Build history of the part. All positions in model axes, mm. Face numbers are marked on the shaded views. A direction names the side the tool comes from. Coordinates: 2 decimals unless noted, no trailing zeros. Order: outer loops, then holes, each group sorted by start corner. A loop starts at its lowest first (then second) coordinate and runs counter-clockwise, first axis right, second up. Notation, with made-up numbers: (80.5, -14.75) - (111.5, -14.75) arc R20 cw to (111.5, 16.25) - close; hole circle Ø4 at (-38, -27.5). An arc over 180 degrees is marked (long way). Answer as CSV lines item,"result". Start each with the question number.
from build123d import *

# Parameters (mm, degrees)
SKETCH1_R           = 8
BOSS_EXTRUDE1_DEPTH = 25
SKETCH2_R           = 5.5
CUT_EXTRUDE1_DEPTH  = 20
SKETCH3_R           = 2.5
CUT_EXTRUDE2_DEPTH  = 6
FILLET1_R           = 0.2
FILLET2_R           = 0.3


with BuildPart() as part:
    # Sketch1 → Boss-Extrude1 (new body)
    with BuildSketch(Plane.XY):
        Circle(SKETCH1_R)
    extrude(amount=BOSS_EXTRUDE1_DEPTH)

    # Sketch2 → Cut-Extrude1 (cut)
    with BuildSketch(Plane.XY.offset(25)):
        Circle(SKETCH2_R)
    extrude(amount=-CUT_EXTRUDE1_DEPTH, mode=Mode.SUBTRACT)

    # Sketch3 → Cut-Extrude2 (cut, through all)
    with BuildSketch(Plane.XY.offset(5)):
        Circle(SKETCH3_R)
    extrude(amount=-CUT_EXTRUDE2_DEPTH, mode=Mode.SUBTRACT)

    # Fillet1
    fillet1_edges = [part.edges().sort_by_distance(p)[0] for p in [
        (-2.5, 0, 0),
        (-2.5, 0, 5),
        (-8, 0, 25),
        (-5.5, 0, 25),
    ]]
    fillet(fillet1_edges, radius=FILLET1_R)

    # Fillet2
    fillet2_edges = [part.edges().sort_by_distance(p)[0] for p in [
        (-8, 0, 0),
    ]]
    fillet(fillet2_edges, radius=FILLET2_R)


solid = part.part
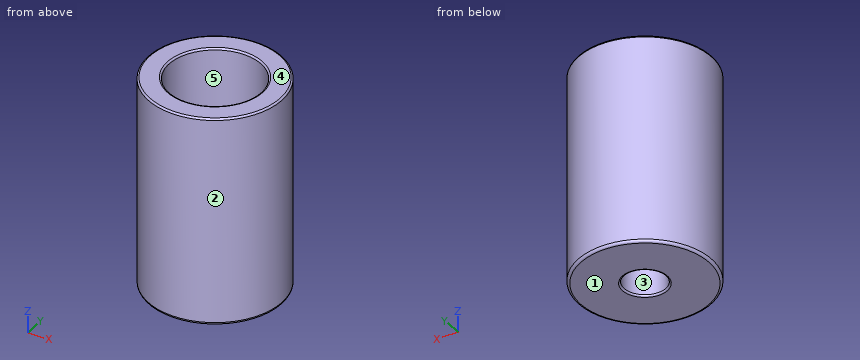
(1) Probe L1, parallel to Y at x = 0, z = 19.75; L2, parallel to Z at x = 3, y = 4.5; L3, parallel to X at y = 3, z = 14.25. List the from-to ranges inside material, lowest first. Write a range as [from, to].
(2) Which spindle directions (+Z, -Z, +X, -X, +Y, -Y) get a long thin tool onto all of the face, cutting with end or side? Do the marked faces 4 and 5. Say none if no direction does.
(3) Band-saw the part on D-D on z = 8.25. List the corners of the cut face in (x, y), plus the area to 3 significant figures.
(4) Band-saw the part on C-C on z = 2.5. List the corners of the cut face in (x, y).
(5) Drop flat-ended pins along their axis: pin 1 Ø5.5 at (x, y) = (-2.5, 1) entering from +Z; pin 2 Ø1 at (y, z) = (-1, 16) entering from -X; pin 3 Ø2 at (y, z) = (4, 5) entering from +X. Give the stop position or say it passes through.
(6) Pull direction X, two halves, no side cores. Call the marked faces 1, 2 and 3: +X half, -X half, draft (parallel to the pull), parting line (faces both ways), or undercut.
(7) Band-saw the part on A-A on x = 0. List the corners of the cut face in (y, z).
Filled in:
1,L1,"y = [-8, -5.5], [5.5, 8]"
1,L2,"z = [0, 5]"
1,L3,"x = [-7.42, -4.61], [4.61, 7.42]"
2,face 4,"+Z, +X, -X, +Y, -Y"
2,face 5,"+Z"
3,outline,"circle Ø16 at (0, 0); hole circle Ø11 at (0, 0)"
3,area,"106 mm^2"
4,outline,"circle Ø16 at (0, 0); hole circle Ø5 at (0, 0)"
5,pin 1,"stops at z = 5"
5,pin 2,"stops at x = -7.98"
5,pin 3,"stops at x = 7.42"
6,face 1,"draft"
6,face 2,"parting line"
6,face 3,"undercut"
7,outline,"(-8, 0.3) arc R0.3 ccw to (-7.7, 0) - (-2.7, 0) arc R0.2 ccw to (-2.5, 0.2) - (-2.5, 4.8) arc R0.2 ccw to (-2.7, 5) - (-5.5, 5) - (-5.5, 24.8) arc R0.2 ccw to (-5.7, 25) - (-7.8, 25) arc R0.2 ccw to (-8, 24.8) - close; (2.5, 0.2) arc R0.2 ccw to (2.7, 0) - (7.7, 0) arc R0.3 ccw to (8, 0.3) - (8, 24.8) arc R0.2 ccw to (7.8, 25) - (5.7, 25) arc R0.2 ccw to (5.5, 24.8) - (5.5, 5) - (2.7, 5) arc R0.2 ccw to (2.5, 4.8) - close"
